from build123d import *

# Parameters (mm, degrees)
SKETCH_1_W          = 17
SKETCH_1_H          = 20
EXTRUDE_1_DEPTH     = 20
SKETCH_2_W          = 12.6
SKETCH_2_H          = 17
CUT_EXTRUDE_1_DEPTH = 17
CUT_EXTRUDE_2_DEPTH = 17
CUT_EXTRUDE_3_DEPTH = 3
CUT_EXTRUDE_4_DEPTH = 3


with BuildPart() as part:
    # 草图1 → 凸台-拉伸1 (new body)
    with BuildSketch(Plane(origin=(0, 0, 0), x_dir=(1, 0, 0), z_dir=(0, 1, 0))):
        Rectangle(SKETCH_1_W, SKETCH_1_H)
    extrude(amount=EXTRUDE_1_DEPTH)

    # 草图2 → 切除-拉伸1 (cut)
    with BuildSketch(Plane(origin=(0, 20, 0), x_dir=(1, 0, 0), z_dir=(0, 1, 0))):
        with Locations((0, -1.5)):
            Rectangle(SKETCH_2_W, SKETCH_2_H)
    extrude(amount=-CUT_EXTRUDE_1_DEPTH, mode=Mode.SUBTRACT)

    # 草图3 → 切除-拉伸2 (cut)
    with BuildSketch(Plane(origin=(8.5, 0, 0), x_dir=(0, 0, -1), z_dir=(1, 0, 0))):
        with BuildLine():
            Line((6, 19), (6, 17))
            Line((6, 17), (-7, 4))
            Line((-7, 4), (-9, 4))
            ThreePointArc((-9, 4), (-9.707106781, 3.707106781), (-10, 3))
            Line((-10, 3), (-10, 20))
            Line((-10, 20), (7, 20))
            ThreePointArc((7, 20), (6.292893219, 19.707106781), (6, 19))
        make_face()
    extrude(amount=-CUT_EXTRUDE_2_DEPTH, mode=Mode.SUBTRACT)

    # 草图4 → 切除-拉伸3 (cut)
    with BuildSketch(Plane.XY.offset(-7)):
        with BuildLine():
            Line((2.9, 11.5), (2.9, 8.5))
            ThreePointArc((2.9, 8.5), (0, 5.6), (-2.9, 8.5))
            Line((-2.9, 8.5), (-2.9, 11.5))
            ThreePointArc((-2.9, 11.5), (0, 14.4), (2.9, 11.5))
        make_face()
    extrude(amount=-CUT_EXTRUDE_3_DEPTH, mode=Mode.SUBTRACT)

    # 草图5 → 切除-拉伸4 (cut)
    with BuildSketch(Plane(origin=(0, 3, 0), x_dir=(1, 0, 0), z_dir=(0, 1, 0))):
        with BuildLine():
            Line((2.9, 1.5), (2.9, -1.5))
            ThreePointArc((2.9, -1.5), (0, -4.4), (-2.9, -1.5))
            Line((-2.9, -1.5), (-2.9, 1.5))
            ThreePointArc((-2.9, 1.5), (0, 4.4), (2.9, 1.5))
        make_face()
    extrude(amount=-CUT_EXTRUDE_4_DEPTH, mode=Mode.SUBTRACT)


solid = part.part
Design review of the part built by this model. Coordinates are the model's own, in mm. A direction names the side the tool comes from. Give positions to 0.01 mm unless a question says otherwise; leave off trailing zeros. Write each loop counter-clockwise with the first axis right and the second up, starting at its lowest first coordinate (ties: lowest second). Pieces come first, ordered by that corner, then holes. Notation, with made-up numbers: M 10.25,78 L 24.25,78 A15 cw 24.25,105 Z; hole C -27.75,84.25 d2. An arc over 180 degrees is marked long. Answer as a JSON object with one key per item and string values. Group by question number.
1) We need section C-C (x = 0). Give the boundary of the cut face in (y, z).
2) Mouldability with a two-part tool opening along Z and no side actions: class faces 4 (the face through (-2.9, 10, -8)), 5 (the face through (-7.385, 19.715, -6.301)), 6 (the face through (2.9, 2, 0)) as released by +Z, released by -Z, zero draft, split by the parting line, or undercut.
3) For line 1 along X through (y, z) = (4.5, 0.75); line 2 along X through (y, z) = (10, -7.5); line 3 along Z through (x, y) = (-5.75, 4), list the stretches that pass through material, from the lowest coordinate up.
4) Clearance check with flat-ended pins moving along their axes: pin 1 Ø1 at (x, z) = (-1.5, 4) entering from +Y; pin 2 Ø2 at (x, z) = (0.5, -0.5) entering from +Y (3 decimals); pin 3 Ø1.6 at (x, y) = (-7, 18) entering from +Z; pin 4 Ø4 at (x, y) = (5, 12) entering from +Z. State where each tip first meets the part, or that it passes through.
5) We need section B-B (y = 9.75). Give the boundary of the cut face in (x, z).
6) Tool access review of faces 1 (the face through (-2.9, 2, 0)), 2 (the face through (6.3, 8, -2)), 3 (the face through (-7, 4, 8)): name each direction out of +Z, -Z, +X, -X, +Y, -Y from which nothing blocks a thin tool from reaching the whole face with its end or side.
7) We need section A-A (z = -0.5). Give the boundary of the cut face in (x, y), and give its area (3 significant figures).
8) We need section D-D (x = 7.25). Give the boundary of the cut face in (y, z), and give its area (3 significant figures).
Answer key:
{
 "1": {"outline": "M 0,-10 L 5.6,-10 L 5.6,-7 L 3,-7 L 3,-4.4 L 0,-4.4 Z; M 0,4.4 L 3,4.4 L 3,10 L 0,10 Z; M 14.4,-10 L 20,-10 L 20,-7 L 14.4,-7 Z"},
 "2": {"face 4": "zero draft", "face 5": "released by +Z", "face 6": "undercut"},
 "3": {"line 1": "x = -8.5 to -6.3, 6.3 to 8.5", "line 2": "x = -8.5 to -2.9, 2.9 to 8.5", "line 3": "z = -10 to -7"},
 "4": {"pin 1": "stops at y = 3", "pin 2": "passes through", "pin 3": "stops at z = -6", "pin 4": "stops at z = 0.52"},
 "5": {"outline": "M -8.5,-10 L -2.9,-10 L -2.9,-7 L -6.3,-7 L -6.3,1.25 L -8.5,1.25 Z; M 2.9,-10 L 8.5,-10 L 8.5,1.25 L 6.3,1.25 L 6.3,-7 L 2.9,-7 Z"},
 "6": {"face 1": "+Y, -Y", "face 2": "+Z, +Y", "face 3": "+Z, +X, -X, +Y"},
 "7": {"outline": "M -8.5,0 L -2.9,0 L -2.9,3 L -6.3,3 L -6.3,11.5 L -8.5,11.5 Z; M 2.9,0 L 8.5,0 L 8.5,11.5 L 6.3,11.5 L 6.3,3 L 2.9,3 Z", "area": "71.0 mm²"},
 "8": {"outline": "M 0,-10 L 20,-10 L 20,-7 A1 ccw 19,-6 L 17,-6 L 4,7 L 4,9 A1 ccw 3,10 L 0,10 Z", "area": "228 mm²"}
}
